```python
from build123d import *

# Parameters (mm, degrees)
F0_W     = 23
F0_H     = 2.6
F1_DEPTH = 9.2
F2_R     = 2.5
F3_DEPTH = 3.1
F4_R     = 2


with BuildPart() as f1:
    # F0 (on Top) → F1 (new body)
    with BuildSketch(Plane.XY):
        Polygon((-39.351552, 9.527253), (-39.351552, 2.727253), (-36.351552, 2.727253), (-36.351552, 4.827253), (-36.351552, 7.427253), (-36.351552, 9.527253), align=None)
        with Locations((-24.851552, 6.127253)):
            Rectangle(F0_W, F0_H)
    extrude(amount=F1_DEPTH)

    # F2 (on face) → F3 (cut)
    with BuildSketch(Plane.XZ.offset(-4.827253)):
        with Locations((-28.351552, 4)):
            Circle(F2_R)
        with Locations((-17.851552, 4)):
            Circle(F2_R)
    extrude(amount=-F3_DEPTH, mode=Mode.SUBTRACT)

    # F4
    f4_edges = [f1.edges().sort_by_distance(p)[0] for p in [
        (-13.351552, 6.127253, 9.2),
    ]]
    fillet(f4_edges, radius=F4_R)


solid = f1.part
```
Check sheet for the modelled part. Datum: model origin and axes. Units: mm. A direction names the side the tool comes from. Give positions to 0.01 mm unless a question says otherwise; leave off trailing zeros. Order: outer loops, then holes, each group sorted by start corner. A loop starts at its lowest first (then second) coordinate and runs counter-clockwise, first axis right, second up. Notation, with made-up numbers: (30, 50.25) -> (37, 50.25) arc R17 cw to (37, 70.25) -> close; hole circle Ø9 at (13, -5). An arc over 180 degrees is marked (long way). Return JSON: item names as keys, results as strings.
1. Cross-section at D-D, the plane z = 4. Record the cut outline in (x, y), plus the area to 3 significant figures.
From the geometry:
{"outline": "(-39.35, 2.73) -> (-36.35, 2.73) -> (-36.35, 4.83) -> (-30.85, 4.83) -> (-30.85, 7.43) -> (-36.35, 7.43) -> (-36.35, 9.53) -> (-39.35, 9.53) -> close; (-25.85, 4.83) -> (-20.35, 4.83) -> (-20.35, 7.43) -> (-25.85, 7.43) -> close; (-15.35, 4.83) -> (-13.35, 4.83) -> (-13.35, 7.43) -> (-15.35, 7.43) -> close", "area": "54.2 mm^2"}
2. Cross-section at C-C, the plane y = 7.75. Record the cut outline in (x, z).
From the geometry:
{"outline": "(-39.35, 0) -> (-36.35, 0) -> (-36.35, 9.2) -> (-39.35, 9.2) -> close"}
3. Cross-section at A-A, the plane z = 3. Record the cut outline in (x, y), plus the area to 3 significant figures.
From the geometry:
{"outline": "(-39.35, 2.73) -> (-36.35, 2.73) -> (-36.35, 4.83) -> (-30.64, 4.83) -> (-30.64, 7.43) -> (-36.35, 7.43) -> (-36.35, 9.53) -> (-39.35, 9.53) -> close; (-26.06, 4.83) -> (-20.14, 4.83) -> (-20.14, 7.43) -> (-26.06, 7.43) -> close; (-15.56, 4.83) -> (-13.35, 4.83) -> (-13.35, 7.43) -> (-15.56, 7.43) -> close", "area": "56.4 mm^2"}
4. Go/stop test with flat-tipped pins: P1, Ø3, axis at x = -26.5, z = 6, coming from the -Y side; P2, Ø2, axis at x = -19.5, y = 3.5, coming from the -Z side; P3, Ø5, axis at x = -30.5, z = 7, coming from the +Y side; P4, Ø1.7, axis at y = 9, z = 4, coming from the +X side. Record where each tip stops, or that it passes through.
From the geometry:
{"P1": "y = 4.83", "P2": "through", "P3": "y = 7.43", "P4": "x = -36.35"}
5. Cross-section at B-B, the plane x = -16. Record the cut outline in (y, z), plus the area to 3 significant figures.
From the geometry:
{"outline": "(4.83, 0) -> (7.43, 0) -> (7.43, 2.32) -> (4.83, 2.32) -> close; (4.83, 5.68) -> (7.43, 5.68) -> (7.43, 9.2) -> (4.83, 9.2) -> close", "area": "15.2 mm^2"}
6. Mould release check, pull along Z, two halves, no side actions. Record for faces 1 (the flat face through (-30, 6, 9.2)), 2 (the flat face through (-29, 6, 0)), 3 (the cylindrical face through (-20.35, 6.11, 4.11)): +Z half, -Z half, draft (parallel to the pull), parting line (faces both ways), or undercut.
From the geometry:
{"face 1": "+Z half", "face 2": "-Z half", "face 3": "undercut"}
7. Set-up check for faces 4 (the flat face through (-36.352, 8, 5)), 5 (the flat face through (-13.352, 6, 4)), 6 (the flat face through (-36.352, 4, 5)): record each of +Z, -Z, +X, -X, +Y, -Y from which the full face is reachable in a straight line by a thin tool's end or side.
From the geometry:
{"face 4": "+Z, -Z, +X, +Y", "face 5": "+Z, -Z, +X, +Y, -Y", "face 6": "+Z, -Z, +X, -Y"}
8. Material ranges on probe 1 along X at (y, z) = (9, 3.75); probe 2 along Y at (x, z) = (-24.5, 2.25); probe 3 along X at (y, z) = (7, 3.5), recorded low to high. Write a range as [from, to].
From the geometry:
{"probe 1": "[-39.35, -36.35]", "probe 2": "[4.83, 7.43]", "probe 3": "[-39.35, -30.8], [-25.9, -20.3], [-15.4, -13.35]"}
